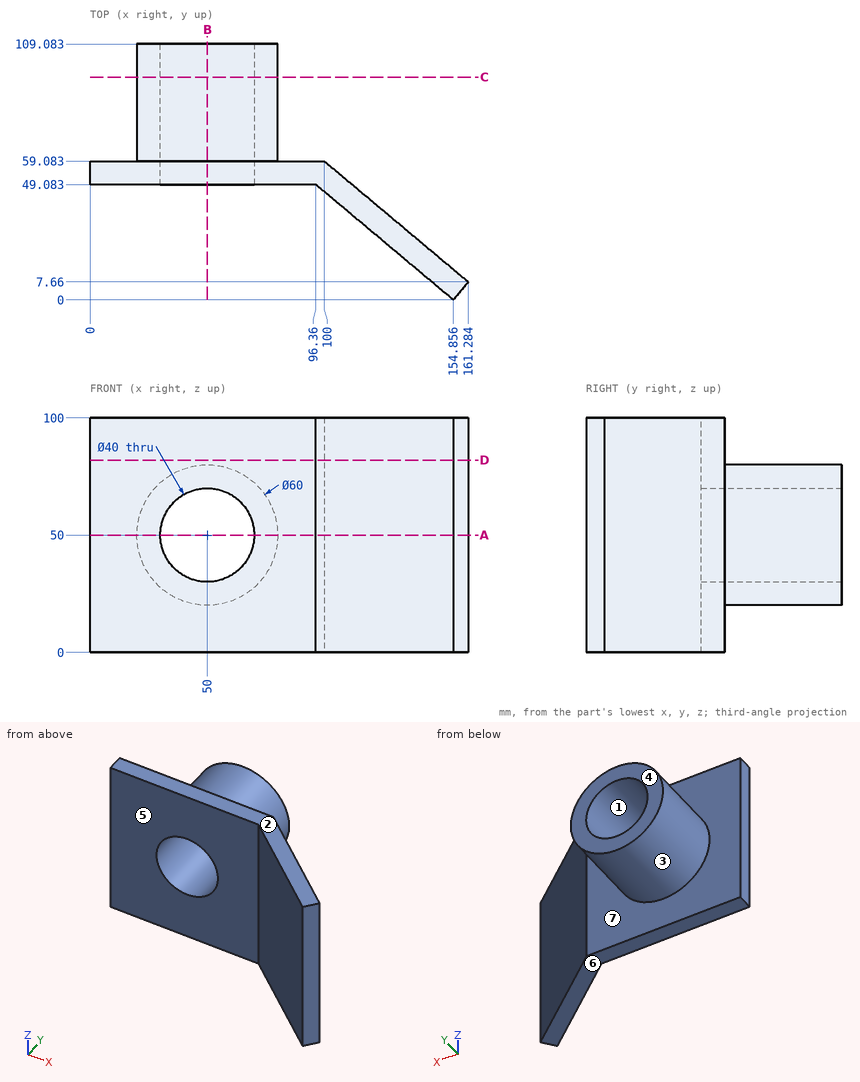
The figure shows three views and two pictorial views of one solid part (mm, origin at its lowest corner). Answer the questions. A direction names the side the tool comes from. Coordinates: 2 decimals unless noted, no trailing zeros. Write each loop counter-clockwise with the first axis right and the second up, starting at its lowest first coordinate (ties: lowest second). Pieces come first, ordered by that corner, then holes. Notation, with made-up numbers: (-34.75, -12) -> (-11.75, -12) arc R16 ccw to (-11.75, 0) -> close; hole circle Ø5 at (18, -15). An arc over 180 degrees is marked (long way). Return JSON: item names as keys, results as strings.
1. Each of these flat-tipped pins is pushed along its axis until it touches: P1, Ø1.5, axis at x = 66.5, z = 67, coming from the -Y side; P2, Ø4, axis at x = 71.5, y = 67, coming from the +Z side; P3, Ø8, axis at x = 58, y = 75, coming from the -Z side. Where does it stop, or does it pass through?
Found:
{"P1": "y = 49.08", "P2": "z = 72.8", "P3": "z = 20.27"}
2. Determine the mould class of the marked faces 1, 2, 3 and 4 for opening direction Z: pulls with the +Z half, pulls with the -Z half, needs draft (parallel to the pull), parting line crosses it, or undercut.
Found:
{"face 1": "undercut", "face 2": "pulls with the +Z half", "face 3": "parting line crosses it", "face 4": "needs draft"}
3. A tool of negligible diameter and unlimited length cuts with its end or side. For the marked faces 5, 6 and 7, from which of +Z, -Z, +X, -X, +Y, -Y can it reach the whole face along a straight path? Write none if from no direction.
Found:
{"face 5": "+Z, -Z, -X, -Y", "face 6": "-Z, +X, -X, +Y, -Y", "face 7": "+Y"}
4. A cutting plane is placed at D-D (z = 82). Determine the outline of the cut face in (x, y) (1 decimal), and give its area (3 significant figures).
Found:
{"outline": "(0, 49.1) -> (96.4, 49.1) -> (154.9, 0) -> (161.3, 7.7) -> (100, 59.1) -> (0, 59.1) -> close", "area": "1,760 mm2"}
5. Find the intervals of material crossed by line 1 along Z through (x, y) = (50, 76.5); line 2 along Y through (x, z) = (85.5, 58), in increasing order. Write a range as from..to.
Found:
{"line 1": "20..30, 70..80", "line 2": "49.08..59.08"}
6. A cutting plane is placed at B-B (x = 50). Determine the outline of the cut face in (y, z).
Found:
{"outline": "(49.08, 0) -> (59.08, 0) -> (59.08, 20) -> (109.08, 20) -> (109.08, 30) -> (49.08, 30) -> close; (49.08, 70) -> (109.08, 70) -> (109.08, 80) -> (59.08, 80) -> (59.08, 100) -> (49.08, 100) -> close"}
7. A cutting plane is placed at C-C (y = 95). Determine the outline of the cut face in (x, z), and give its area (3 significant figures).
Found:
{"outline": "circle Ø60 at (50, 50); hole circle Ø40 at (50, 50)", "area": "1,570 mm2"}
8. A cutting plane is placed at A-A (z = 50). Determine the outline of the cut face in (x, y) (1 decimal), and give its area (3 significant figures).
Found:
{"outline": "(0, 49.1) -> (30, 49.1) -> (30, 109.1) -> (20, 109.1) -> (20, 59.1) -> (0, 59.1) -> close; (70, 49.1) -> (96.4, 49.1) -> (154.9, 0) -> (161.3, 7.7) -> (100, 59.1) -> (80, 59.1) -> (80, 109.1) -> (70, 109.1) -> close", "area": "2,360 mm2"}
